from build123d import *
from build123d.topology import SkipClean

# Parameters (mm, degrees)
CUT_EXTRUDE1_DEPTH       = 1.04902
CIRPATTERN1_COUNT        = 6
CIRPATTERN1_COPY_1_DEPTH = 1.04902
CIRPATTERN1_COPY_2_DEPTH = 1.04902
CIRPATTERN1_COPY_3_DEPTH = 1.04902
CIRPATTERN1_COPY_4_DEPTH = 1.04902
CIRPATTERN1_COPY_5_DEPTH = 1.04902


with BuildPart() as part:
    # Sketch2 → Revolve1 (revolve)
    with BuildSketch(Plane(origin=(0, 0, 0), x_dir=(0, 0, -1), z_dir=(1, 0, 0))):
        Polygon((1.4986, 1.4224), (4.19735, 1.4224), (4.6736, 0.94615), (4.6736, 0), (1.4986, 0), align=None)
    revolve(axis=Axis((0, 0, -4.6736), (0, 0, 1)))


with BuildPart() as body_2:
    # Sketch3 → Revolve2 (revolve)
    with BuildSketch(Plane(origin=(0, 0, 0), x_dir=(0, 0, -1), z_dir=(1, 0, 0)), mode=Mode.PRIVATE) as revolve2_sk:
        with BuildLine():
            Line((1.4986, 0), (1.4986, 2.7051))
            Line((1.4986, 2.7051), (1.27381, 2.7051))
            ThreePointArc((1.27381, 2.7051), (0.543126817, 2.17424602), (0, 1.4526387))
            Line((0, 1.4526387), (0, 0))
            Line((0, 0), (1.4986, 0))
        make_face()
    revolve(revolve2_sk.sketch.rotate(Axis((0, 0, 0), (0, 0, -1)), 90), axis=Axis((0, 0, 0), (0, 0, -1)))

    # Combine1: union part
    add(part.part)

    # Sketch4 → Cut-Extrude1 (cut)
    with BuildSketch(Plane.XY):
        with BuildLine():
            Line((-0.886596525, 0), (0, 0))
            Line((0, 0), (-1.023753485, 0.59106435))
            ThreePointArc((-1.023753485, 0.59106435), (-1.035216975, 0.548031955), (-1.023503515, 0.505066928))
            ThreePointArc((-1.023503515, 0.505066928), (-0.921429906, 0.261646769), (-0.886596525, 0))
        make_face()
    cut_extrude1 = extrude(amount=-CUT_EXTRUDE1_DEPTH, mode=Mode.SUBTRACT)

    # Mirror1: Cut-Extrude1 across plane
    add(cut_extrude1.mirror(Plane.ZX), mode=Mode.SUBTRACT)

    # CirPattern1: Cut-Extrude1 ×6 about axis
    cirpattern1_axis = Axis((0, 0, 0), (0, 0, 1))
    for i in range(1, CIRPATTERN1_COUNT):
        add(cut_extrude1.rotate(cirpattern1_axis, i * 360 / CIRPATTERN1_COUNT), mode=Mode.SUBTRACT)

    # CirPattern1 copy 1 sketch → CirPattern1 copy 1 (cut)
    with BuildSketch(Plane(origin=(0, 0, 0), x_dir=(0.5000000000000001, 0.8660254037844386, 0), z_dir=(0, 0, 1))):
        with BuildLine():
            Line((-0.886596525, 0), (0, 0))
            Line((0, 0), (-1.023753485, -0.59106435))
            ThreePointArc((-1.023753485, -0.59106435), (-1.035216975, -0.548031955), (-1.023503515, -0.505066928))
            ThreePointArc((-1.023503515, -0.505066928), (-0.921429906, -0.261646769), (-0.886596525, 0))
        make_face()
    extrude(amount=-CIRPATTERN1_COPY_1_DEPTH, mode=Mode.SUBTRACT)

    # CirPattern1 copy 2 sketch → CirPattern1 copy 2 (cut)
    with BuildSketch(Plane(origin=(0, 0, 0), x_dir=(-0.4999999999999998, 0.8660254037844387, 0), z_dir=(0, 0, 1))):
        with BuildLine():
            Line((-0.886596525, 0), (0, 0))
            Line((0, 0), (-1.023753485, -0.59106435))
            ThreePointArc((-1.023753485, -0.59106435), (-1.035216975, -0.548031955), (-1.023503515, -0.505066928))
            ThreePointArc((-1.023503515, -0.505066928), (-0.921429906, -0.261646769), (-0.886596525, 0))
        make_face()
    extrude(amount=-CIRPATTERN1_COPY_2_DEPTH, mode=Mode.SUBTRACT)

    # CirPattern1 copy 3 sketch → CirPattern1 copy 3 (cut)
    with BuildSketch(Plane(origin=(0, 0, 0), x_dir=(-1, 0, 0), z_dir=(0, 0, 1))):
        with BuildLine():
            Line((-0.886596525, 0), (0, 0))
            Line((0, 0), (-1.023753485, -0.59106435))
            ThreePointArc((-1.023753485, -0.59106435), (-1.035216975, -0.548031955), (-1.023503515, -0.505066928))
            ThreePointArc((-1.023503515, -0.505066928), (-0.921429906, -0.261646769), (-0.886596525, 0))
        make_face()
    extrude(amount=-CIRPATTERN1_COPY_3_DEPTH, mode=Mode.SUBTRACT)

    # CirPattern1 copy 4 sketch → CirPattern1 copy 4 (cut)
    with BuildSketch(Plane(origin=(0, 0, 0), x_dir=(-0.5000000000000004, -0.8660254037844384, 0), z_dir=(0, 0, 1))):
        with BuildLine():
            Line((-0.886596525, 0), (0, 0))
            Line((0, 0), (-1.023753485, -0.59106435))
            ThreePointArc((-1.023753485, -0.59106435), (-1.035216975, -0.548031955), (-1.023503515, -0.505066928))
            ThreePointArc((-1.023503515, -0.505066928), (-0.921429906, -0.261646769), (-0.886596525, 0))
        make_face()
    extrude(amount=-CIRPATTERN1_COPY_4_DEPTH, mode=Mode.SUBTRACT)

    # CirPattern1 copy 5 sketch → CirPattern1 copy 5 (cut)
    with BuildSketch(Plane(origin=(0, 0, 0), x_dir=(0.5000000000000001, -0.8660254037844386, 0), z_dir=(0, 0, 1))):
        with BuildLine():
            Line((-0.886596525, 0), (0, 0))
            Line((0, 0), (-1.023753485, -0.59106435))
            ThreePointArc((-1.023753485, -0.59106435), (-1.035216975, -0.548031955), (-1.023503515, -0.505066928))
            ThreePointArc((-1.023503515, -0.505066928), (-0.921429906, -0.261646769), (-0.886596525, 0))
        make_face()
    extrude(amount=-CIRPATTERN1_COPY_5_DEPTH, mode=Mode.SUBTRACT)

    # Sketch5 → Cut-Revolve1 (revolve, cut)
    with SkipClean():  # the faces are left unmerged after this step: merging them gives an invalid solid
        with BuildSketch(Plane(origin=(0, 0, 0), x_dir=(0, 0, -1), z_dir=(1, 0, 0))):
            with BuildLine():
                Line((-2.159882457, 2.50955579), (-2.159882457, -2.50955579))
                ThreePointArc((-2.159882457, -2.50955579), (0.349673333, 0), (-2.159882457, 2.50955579))
            make_face()
        revolve(axis=Axis((0, 2.50955579, 2.159882457), (0, -1, 0)), mode=Mode.SUBTRACT)


solid = body_2.part
Work out the finished part from the listing and answer in its coordinate system (mm). Coordinates: 2 decimals unless noted, no trailing zeros. Write each loop counter-clockwise with the first axis right and the second up, starting at its lowest first coordinate (ties: lowest second). Pieces come first, ordered by that corner, then holes. Notation, with made-up numbers: M 3,-2 L 18,-2 A13 cw 18,8 Z; hole C -13.5,45 d8. An arc over 180 degrees is marked long. Use one line per item in the form item = value. Start each with the question number.
1. The mould has two halves that part along X. Classify faces 1 (the face through (0, 0, -1.049)), 2 (the face through (-1.2, 1.2, -1.499)), 3 (the face through (1.39, -0.31, -2.87)): released by +X, released by -X, zero draft, split by the parting line, or undercut.
2. This flat-tipped pin is pushed along its axis until it touches: P1, Ø1.5, axis at y = 1, z = -4, coming from the +X side. Where does it stop, or does it pass through?
3. Straight lines are drawn through the part: probe 1 along X at (y, z) = (0.05, -3.5); probe 2 along Z at (x, y) = (2.2, 0.3). For each, find the intervals that lie inside material, in ascending order. Write a range as from..to.
4. The part is cut by section B-B (y = -2.1). Give the vertices of the cut face in (x, z).
5. The part is cut by section A-A (z = -0.45). Give the vertices of the cut face in (x, y), plus the area to 3 significant figures.
6. The part is cut by section C-C (x = 1.75). Give the vertices of the cut face in (y, z).
7. The part is cut by section D-D (z = -3.8). Give the vertices of the cut face in (x, y).
Evaluation:
q1.face_1 = undercut
q1.face_2 = zero draft
q1.face_3 = split by the parting line
q2.P1 = 1.4
q3.probe_1 = -1.42..1.42
q3.probe_2 = -1.5..-0.59
q4.outline = M -1.71,-1.5 L 1.71,-1.5 L 1.71,-1.27 A2.21 ccw -1.71,-1.27 Z
q5.outline = C 0,0 d4.16; hole M -1.02,-0.51 A0.09 ccw -0.95,-0.63 A1 cw -0.07,-1.14 A0.09 ccw 0.07,-1.14 A1 cw 0.95,-0.63 A0.09 ccw 1.02,-0.51 A1 cw 1.02,0.51 A0.09 ccw 0.95,0.63 A1 cw 0.07,1.14 A0.09 ccw -0.07,1.14 A1 cw -0.95,0.63 A0.09 ccw -1.02,0.51 A1 cw Z
q5.area = 10.5 mm^2
q6.outline = M -2.06,-1.5 L 2.06,-1.5 L 2.06,-1.27 A2.5 ccw -2.06,-1.27 Z
q7.outline = C 0,0 d2.84
